The listing builds one solid part. Answer for the finished solid, in the listing's coordinates (mm). Round coordinates to 2 decimals unless told otherwise and drop trailing zeros. Loops run counter-clockwise (first coordinate to the right, second up) from the corner with the lowest first, then second, coordinate; pieces in that order, holes last. Notation, with made-up numbers: (28, -10.5) - (64, -10.5) arc R28 ccw to (64, 17.5) - close; hole circle Ø1 at (66, 72.25). An arc over 180 degrees is marked (long way). Write item = value, one per line. Start each with the question number.
1) Given pin 1 Ø1 at (x, y) = (3.5, -6.5) entering from -Z; pin 2 Ø1.5 at (x, y) = (-29.5, -1) entering from -Z, each flat-ended and moving along its own axis, determine where each tip first touches the part or whether it passes through.
2) Section A-A, the plane y = -5.5 is taken. Determine the outline of the cut face in (x, z).
3) Straight lines are drawn through the part: line 1 along Z through (x, y) = (3.5, -4.5); line 2 along Z through (x, y) = (-30, -1.25); line 3 along X through (y, z) = (-5.75, 3). For each, find the intervals that lie inside material, in ascending order.
from build123d import *

# Parameters (mm, degrees)
F1_DEPTH = 7.3
F2_R     = 3


with BuildPart() as f1:
    # F0 (on Front) → F1 (new body)
    with BuildSketch(Plane.XZ):
        with BuildLine():
            Line((29.231137, 79.1), (-29.231137, 79.1))
            ThreePointArc((-29.231137, 79.1), (-36.103411, 76.253411), (-38.95, 69.381137))
            Line((-38.95, 69.381137), (-38.95, -69.381137))
            ThreePointArc((-38.95, -69.381137), (-36.103411, -76.253411), (-29.231137, -79.1))
            Line((-29.231137, -79.1), (29.231137, -79.1))
            ThreePointArc((29.231137, -79.1), (36.103411, -76.253411), (38.95, -69.381137))
            Line((38.95, -69.381137), (38.95, 69.381137))
            ThreePointArc((38.95, 69.381137), (36.103411, 76.253411), (29.231137, 79.1))
        make_face()
    extrude(amount=F1_DEPTH)

    # F2
    f2_edges = [f1.edges().sort_by_distance(p)[0] for p in [
        (38.95, -7.3, 0),
        (36.103411, -7.3, 76.253411),
        (0, -7.3, 79.1),
        (-36.103411, -7.3, 76.253411),
        (-38.95, -7.3, 0),
        (-36.103411, -7.3, -76.253411),
        (0, -7.3, -79.1),
        (36.103411, -7.3, -76.253411),
        (38.95, 0, 0),
        (36.103411, 0, 76.253411),
        (0, 0, 79.1),
        (-36.103411, 0, 76.253411),
        (-38.95, 0, 0),
        (-36.103411, 0, -76.253411),
        (0, 0, -79.1),
        (36.103411, 0, -76.253411),
    ]]
    fillet(f2_edges, radius=F2_R)


solid = f1.part
Geometry check:
q1.pin_1 = -78.57
q1.pin_2 = -78.82
q2.outline = (-38.7, -69.38) arc R9.47 ccw to (-29.23, -78.85) - (29.23, -78.85) arc R9.47 ccw to (38.7, -69.38) - (38.7, 69.38) arc R9.47 ccw to (29.23, 78.85) - (-29.23, 78.85) arc R9.47 ccw to (-38.7, 69.38) - close
q3.line_1 = -79.09 to 79.09
q3.line_2 = -78.5 to 78.5
q3.line_3 = -38.58 to 38.58
